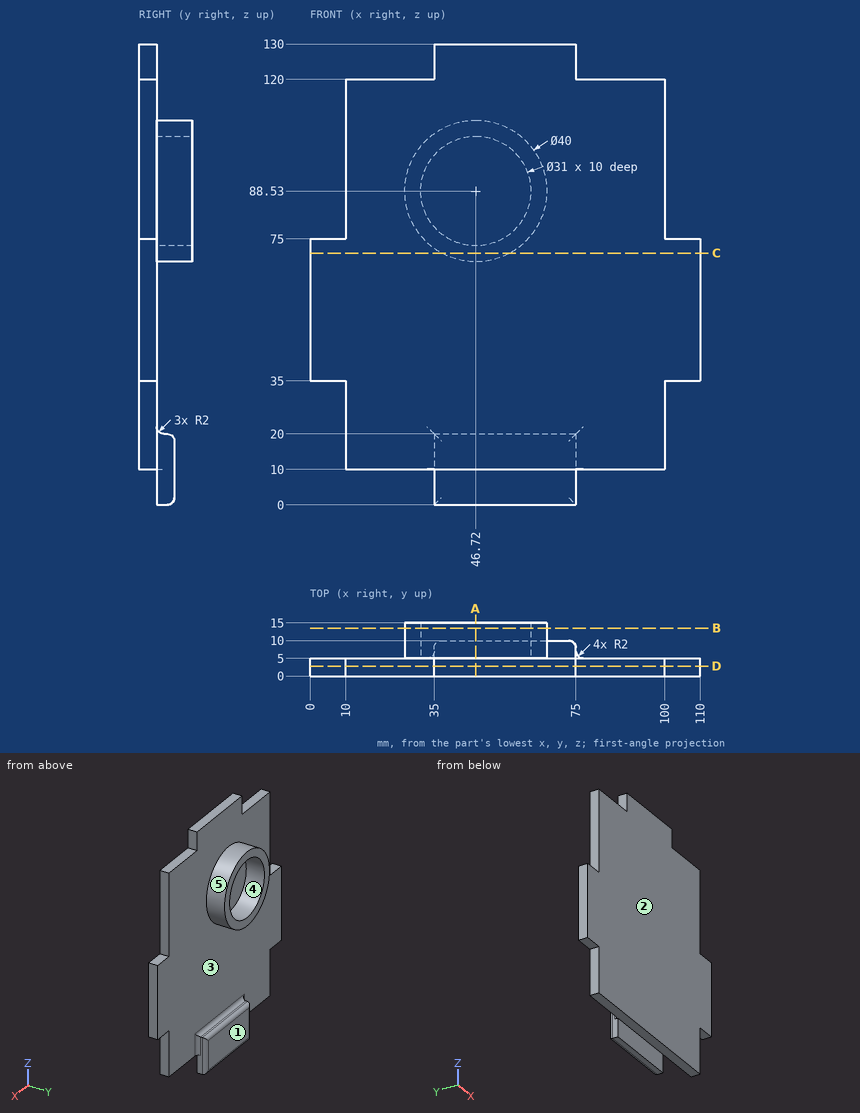
For this review, use the dimensioned drawing (mm, ordinates from the lowest corner) and the shaded views. A direction names the side the tool comes from. Round coordinates to 2 decimals unless told otherwise and drop trailing zeros. Order: outer loops, then holes, each group sorted by start corner. A loop starts at its lowest first (then second) coordinate and runs counter-clockwise, first axis right, second up. Notation, with made-up numbers: (78, 76) -> (103, 76) arc R10 ccw to (103, 91) -> close; hole circle Ø10 at (32.25, 75). An arc over 180 degrees is marked (long way). One line per item, written item: value. Start each with the question number.
Q1. Take a section at D-D (y = 2.75). Write out the cut boundary in (x, z), and give its area (3 significant figures).
Q2. Take a section at B-B (y = 13.5). Write out the cut boundary in (x, z), and give its area (3 significant figures).
Q3. Wall thickness on line 1 (X direction, y = 13.25, z = 88.53); line 2 (Y direction, x = 46, z = 80); line 3 (Z direction, x = 97, y = 3): over which ranges is each line inside the solid? List them lowest first.
Q4. Take a section at A-A (x = 46.72). Write out the cut boundary in (y, z).
Q5. Mouldability with a two-part tool opening along X and no side actions: class the marked faces 3, 4 and 5 as released by +X, released by -X, zero draft, split by the parting line, or undercut.
Q6. Take a section at C-C (z = 71). Write out the cut boundary in (x, y).
Q7. Clearance check with flat-ended pins moving along their axes: pin 1 Ø5.5 at (x, y) = (25.5, 3) entering from +Z; pin 2 Ø2.5 at (x, y) = (105, 1.5) entering from +Z; pin 3 Ø5.5 at (y, z) = (3.5, 90) entering from +X. State where each tip first meets the part, or that it passes through.
Q8. Machinability: for the marked faces 1 and 2, which of the approach directions +Z, -Z, +X, -X, +Y, -Y give a long, thin tool a straight path to every point of the face, cutting with its end or side? Answer none if there is none.
Reported:
1. outline: (0, 35) -> (10, 35) -> (10, 10) -> (100, 10) -> (100, 35) -> (110, 35) -> (110, 75) -> (100, 75) -> (100, 120) -> (75, 120) -> (75, 130) -> (35, 130) -> (35, 120) -> (10, 120) -> (10, 75) -> (0, 75) -> close
1. area: 11,100 mm2
2. outline: circle Ø40 at (46.72, 88.53); hole circle Ø31 at (46.72, 88.53)
2. area: 502 mm2
3. line 1: x = 26.72 to 31.22, 62.22 to 66.72
3. line 2: y = 0 to 5
3. line 3: z = 10 to 120
4. outline: (0, 10) -> (5, 10) -> (5, 0) -> (8, 0) arc R2 ccw to (10, 2) -> (10, 18) arc R2 ccw to (8, 20) -> (7, 20) arc R2 cw to (5, 22) -> (5, 68.53) -> (15, 68.53) -> (15, 73.03) -> (5, 73.03) -> (5, 104.03) -> (15, 104.03) -> (15, 108.53) -> (5, 108.53) -> (5, 130) -> (0, 130) -> close
5. face 3: zero draft
5. face 4: undercut
5. face 5: split by the parting line
6. outline: (0, 0) -> (110, 0) -> (110, 5) -> (56.35, 5) -> (56.35, 15) -> (37.09, 15) -> (37.09, 5) -> (0, 5) -> close
7. pin 1: stops at z = 120
7. pin 2: stops at z = 75
7. pin 3: stops at x = 100
8. face 1: -Z, +X, -X, +Y
8. face 2: +Z, -Z, +X, -X, -Y
